Autodesk Inventor part; units mm, degrees
ref_plane "YZ Plane" through (0, 0, 0) normal (1, 0, 0) x (0, 1, 0)
ref_plane "XZ Plane" through (0, 0, 0) normal (0, 1, 0) x (-1, 0, 0)
ref_plane "XY Plane" through (0, 0, 0) normal (0, 0, 1) x (1, 0, 0)
sketch "Sketch1" plane through (0, 0, 0) normal (0, 1, 0) x (-1, 0, 0)
  line L0 (0, 0) -> (-20, 0)
  line L1 (-20, 0) -> (-20, -50)
  line L2 (-20, -50) -> (0, -50)
  line L3 (0, -50) -> (0, 0)
  circle A0 centre (-10, -10.0524) radius 2.5
  circle A1 centre (-10, -37.2673) radius 2.5
  dimension "d0" = 20
  dimension "d1" = 50
  dimension "d2" = 5
  dimension "d3" = 5
extrude "Extrusion1" add sketch "Sketch1" along normal blind 3
sketch "Sketch2" plane through (0, 0, 0) normal (0, 0, 1) x (1, 0, 0)
  line L0 (0, 0) -> (20, 0)
  line L1 (20, 0) -> (20, 100)
  line L2 (20, 100) -> (0, 100)
  line L3 (0, 100) -> (0, 0)
  circle A0 centre (10, 90.706) radius 2.55
  dimension "d6" = 20
  dimension "d7" = 100
  dimension "d8" = 5.1
  dimension "d9" = 90.706
extrude "Extrusion2" add sketch "Sketch2" along normal blind 3
fillet "Fillet1" radius 5 2 edges at (20, 1.5, -50) (0, 1.5, -50)
fillet "Fillet2" radius 5 2 edges at (20, 100, 1.5) (0, 100, 1.5)
properties part number "support bar"
Work out the finished part from the listing and answer in its coordinate system (mm). A direction names the side the tool comes from. Round coordinates to 2 decimals unless told otherwise and drop trailing zeros. Write each loop counter-clockwise with the first axis right and the second up, starting at its lowest first coordinate (ties: lowest second). Pieces come first, ordered by that corner, then holes. Notation, with made-up numbers: (36, 7.5) -> (50, 7.5) arc R16 ccw to (50, 38.5) -> close; hole circle Ø3 at (7.5, -29.5). An arc over 180 degrees is marked (long way). Write each question's results on one line, items separated by ' | '.
Q1. Section D-D, the plane x = 17.75 is taken. Write down the section's boundary in (y, z).
Data:
outline: (0, -49.18) -> (3, -49.18) -> (3, 0) -> (99.18, 0) -> (99.18, 3) -> (0, 3) -> close
Q2. Determine the mould class of faces 1 (the flat face through (20, 33.2, 0.4)), 2 (the flat face through (10, 51, 3)), 3 (the cylindrical face through (10.542, 1.479, -34.827)) for opening direction X: released by +X, released by -X, zero draft, split by the parting line, or undercut.
Data:
face 1: released by +X | face 2: zero draft | face 3: undercut
Q3. Section A-A, the plane x = 10 is taken. Write down the section's boundary in (y, z).
Data:
outline: (0, -50) -> (3, -50) -> (3, -39.77) -> (0, -39.77) -> close; (0, -34.77) -> (3, -34.77) -> (3, -12.55) -> (0, -12.55) -> close; (0, -7.55) -> (3, -7.55) -> (3, 0) -> (88.16, 0) -> (88.16, 3) -> (0, 3) -> close; (93.26, 0) -> (100, 0) -> (100, 3) -> (93.26, 3) -> close
Q4. Which of the six approach directions +Z, -Z, +X, -X, +Y, -Y give full straight-line access (tool end or side, diameter ignored) to faces 4 (the flat face through (10, 3, -25)), 5 (the flat face through (0, 33.2, 0.2))?
Data:
face 4: -Z, +X, -X, +Y | face 5: +Z, -Z, -X, +Y, -Y
Q5. Section B-B, the plane y = 21 is taken. Write down the section's boundary in (x, z).
Data:
outline: (0, 0) -> (20, 0) -> (20, 3) -> (0, 3) -> close
Q6. Straight lines are drawn through the part: line 1 along Z through (x, y) = (10, 2.1); line 2 along Y through (x, z) = (10, 0.8); line 3 along Y through (x, z) = (16.5, -44.5). For each, find the intervals that lie inside material, in ascending order. Write a range as [from, to].
Data:
line 1: [-50, -39.77], [-34.77, -12.55], [-7.55, 3] | line 2: [0, 88.16], [93.26, 100] | line 3: [0, 3]
Q7. Flat-ended cylindrical pins translate along their axes: P1, Ø4.5, axis at x = 10, z = -10.05, coming from the -Y side; P2, Ø3, axis at x = 14.5, z = -14, coming from the +Y side; P3, Ø8, axis at x = 10, z = -37.27, coming from the -Y side. Find the tip coordinate at first contact, or state that the pin passes through.
Data:
P1: through | P2: y = 3 | P3: y = 0
